from build123d import *

# Parameters (mm, degrees)
SKETCH1_R           = 42.5
BOSS_EXTRUDE1_DEPTH = 10
SKETCH2_R           = 1.5
CUT_EXTRUDE1_DEPTH  = 5
SKETCH3_R           = 2.25
CUT_EXTRUDE2_DEPTH  = 11
SKETCH4_R           = 5
CUT_EXTRUDE3_DEPTH  = 4.4
SKETCH5_R           = 2
CUT_EXTRUDE4_DEPTH  = 11


with BuildPart() as part:
    # Sketch1 → Boss-Extrude1 (new body)
    with BuildSketch(Plane(origin=(0, 0, 0), x_dir=(1, 0, 0), z_dir=(0, 1, 0))):
        Circle(SKETCH1_R)
    extrude(amount=BOSS_EXTRUDE1_DEPTH)

    # Sketch2 → Cut-Extrude1 (cut)
    with BuildSketch(Plane(origin=(0, 10, 0), x_dir=(1, 0, 0), z_dir=(0, 1, 0))):
        with Locations((-22.5, 0)):
            Circle(SKETCH2_R)
        with Locations((22.5, 0)):
            Circle(SKETCH2_R)
    extrude(amount=-CUT_EXTRUDE1_DEPTH, mode=Mode.SUBTRACT)

    # Sketch3 → Cut-Extrude2 (cut, through all)
    with BuildSketch(Plane(origin=(0, 10, 0), x_dir=(1, 0, 0), z_dir=(0, 1, 0))):
        with Locations((0, 22)):
            Circle(SKETCH3_R)
        with Locations((19.052558883, -11)):
            Circle(SKETCH3_R)
        with Locations((-19.052558883, -11)):
            Circle(SKETCH3_R)
    extrude(amount=-CUT_EXTRUDE2_DEPTH, mode=Mode.SUBTRACT)

    # Sketch4 → Cut-Extrude3 (cut)
    with BuildSketch(Plane.XZ):
        with Locations((0, -22)):
            Circle(SKETCH4_R)
        with Locations((19.052558883, 11)):
            Circle(SKETCH4_R)
        with Locations((-19.052558883, 11)):
            Circle(SKETCH4_R)
    extrude(amount=-CUT_EXTRUDE3_DEPTH, mode=Mode.SUBTRACT)

    # Sketch5 → Cut-Extrude4 (cut, through all)
    with BuildSketch(Plane(origin=(0, 10, 0), x_dir=(1, 0, 0), z_dir=(0, 1, 0))):
        with Locations((-7.5, 18.5)):
            Circle(SKETCH5_R)
        with Locations((7.5, 18.5)):
            Circle(SKETCH5_R)
    extrude(amount=-CUT_EXTRUDE4_DEPTH, mode=Mode.SUBTRACT)


solid = part.part
Design review of the part built by this model. Coordinates are the model's own, in mm. A direction names the side the tool comes from. Give positions to 0.01 mm unless a question says otherwise; leave off trailing zeros. Loops run counter-clockwise (first coordinate to the right, second up) from the corner with the lowest first, then second, coordinate; pieces in that order, holes last. Notation, with made-up numbers: M 39,58.5 L 70,58.5 A26 ccw 70,85.5 Z; hole C -7.5,78.25 d5. An arc over 180 degrees is marked long. Answer as a JSON object with one key per item and string values.
Item 1: For P1, Ø3, axis at x = -20, z = 13, coming from the -Y side; P2, Ø1, axis at y = 2.5, z = -12, coming from the -X side; P3, Ø0.9, axis at x = -22, z = 0, coming from the +Y side; P4, Ø4.5, axis at x = 7.5, z = -18.5, coming from the -Y side, all flat-tipped, find the tip position at first contact; note any pin that passes through.
Output values:
{"P1": "stops at y = 4.4", "P2": "stops at x = -40.91", "P3": "stops at y = 5", "P4": "stops at y = 0"}
Item 2: We need section B-B (y = 8.5). State the section outline as (x, z) points, and give its area (3 significant figures).
Output values:
{"outline": "C 0,0 d85; hole C -22.5,0 d3; hole C -19.05,11 d4.5; hole C -7.5,-18.5 d4; hole C 0,-22 d4.5; hole C 7.5,-18.5 d4; hole C 19.05,11 d4.5; hole C 22.5,0 d3", "area": "5,590 mm2"}
Item 3: Wall thickness on line 1 along X through (y, z) = (7.3, 0); line 2 along X through (y, z) = (9.25, 11); line 3 along Z through (x, y) = (21.5, 4): over which ranges is each line inside the solid? List them lowest first.
Output values:
{"line 1": "x = -42.5 to -24, -21 to 21, 24 to 42.5", "line 2": "x = -41.05 to -21.3, -16.8 to 16.8, 21.3 to 41.05", "line 3": "z = -36.66 to 6.64, 15.36 to 36.66"}
Item 4: We need section D-D (z = 11). State the section outline as (x, y) points, and give its area (3 significant figures).
Output values:
{"outline": "M -41.05,0 L -24.05,0 L -24.05,4.4 L -21.3,4.4 L -21.3,10 L -41.05,10 Z; M -16.8,4.4 L -14.05,4.4 L -14.05,0 L 14.05,0 L 14.05,4.4 L 16.8,4.4 L 16.8,10 L -16.8,10 Z; M 21.3,4.4 L 24.05,4.4 L 24.05,0 L 41.05,0 L 41.05,10 L 21.3,10 Z", "area": "683 mm2"}
Item 5: Mouldability with a two-part tool opening along Z and no side actions: class faces 4 (the face through (-33.727, 4.93, 25.861)), 5 (the face through (17.394, 7.239, 9.479)), 6 (the face through (-1, 0, -1)) as pulls with the +Z half, pulls with the -Z half, needs draft (parallel to the pull), parting line crosses it, or undercut.
Output values:
{"face 4": "parting line crosses it", "face 5": "undercut", "face 6": "needs draft"}
Item 6: Machinability: for faces 1 (the face through (-0.488, 7.239, -19.804)), 2 (the face through (-23, 5, 0)), 3 (the face through (23.822, 2.169, 12.502)), which of the approach directions +Z, -Z, +X, -X, +Y, -Y give a long, thin tool a straight path to every point of the face, cutting with its end or side? Answer none if there is none.
Output values:
{"face 1": "+Y, -Y", "face 2": "+Y", "face 3": "-Y"}
Item 7: We need section C-C (x = 7). State the section outline as (y, z) points, and give its area (3 significant figures).
Output values:
{"outline": "M 0,-41.92 L 10,-41.92 L 10,-20.44 L 0,-20.44 Z; M 0,-16.56 L 10,-16.56 L 10,41.92 L 0,41.92 Z", "area": "800 mm2"}
Item 8: We need section A-A (z = 0). State the section outline as (x, y) points.
Output values:
{"outline": "M -42.5,0 L 42.5,0 L 42.5,10 L 24,10 L 24,5 L 21,5 L 21,10 L -21,10 L -21,5 L -24,5 L -24,10 L -42.5,10 Z"}
